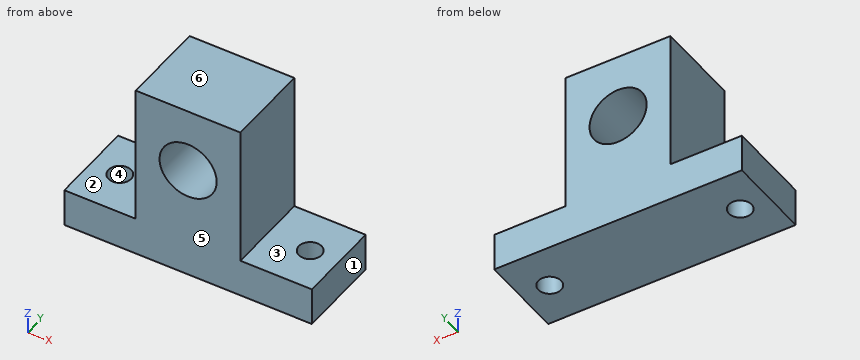
from build123d import *

# Parameters (mm, degrees)
F0_W     = 17.4625
F0_H     = 23.495
F0_R     = 4.7625
F1_DEPTH = 14.2875
F3_D     = 3.7973


with BuildPart() as f1:
    # F0 (on Front) → F1 (new body)
    with BuildSketch(Plane.XZ):
        with Locations((0, 14.9225)):
            Rectangle(F0_W, F0_H)
        with Locations((0, 15.875)):
            Circle(F0_R, mode=Mode.SUBTRACT)
        Polygon((20.6375, -3.175), (20.6375, 3.175), (8.73125, 3.175), (-8.73125, 3.175), (-20.6375, 3.175), (-20.6375, -3.175), align=None)
    extrude(amount=F1_DEPTH)

    # F3 (through all)
    with Locations(Plane(origin=(0, 0, -3.175), x_dir=(1, 0, 0), z_dir=(0, 0, -1))):
        with Locations((-15.875, 7.14375), (15.875, 7.14375)):
            Hole(F3_D / 2)


solid = f1.part
Can you work these out from the model? Positions are in its coordinate system, mm. Face numbers are marked on the shaded views. A direction names the side the tool comes from. Round coordinates to 2 decimals unless told otherwise and drop trailing zeros. Order: outer loops, then holes, each group sorted by start corner. A loop starts at its lowest first (then second) coordinate and runs counter-clockwise, first axis right, second up. Notation, with made-up numbers: (68.25, 53.5) - (119.25, 53.5) arc R16 cw to (119.25, 57.5) - close; hole circle Ø6 at (83, 25.5). An arc over 180 degrees is marked (long way). Answer in a Markdown table with one row per item.
(1) For P1, Ø1, axis at y = -7.5, z = 15.5, coming from the +X side, with a flat end and sliding along its axis, tell me the tip position at first contact or that it passes through.
From the geometry:
| item | result |
|---|---|
| P1 | stops at x = 8.73 |
(2) Suppose I cut it at C-C, the plane y = -11.75. Please give me the cut outline in (x, z) (1 decimal), plus the area to 3 significant figures.
From the geometry:
| item | result |
|---|---|
| outline | (-20.6, -3.2) - (20.6, -3.2) - (20.6, 3.2) - (8.7, 3.2) - (8.7, 26.7) - (-8.7, 26.7) - (-8.7, 3.2) - (-20.6, 3.2) - close; hole circle Ø9.5 at (0, 15.9) |
| area | 601 mm2 |
(3) Which directions (+Z, -Z, +X, -X, +Y, -Y) give clear straight access to the entire face, cutting with the end or side of a thin tool? Please do the marked faces 1, 2 and 3.
From the geometry:
| item | result |
|---|---|
| face 1 | +Z, -Z, +X, +Y, -Y |
| face 2 | +Z, -X, +Y, -Y |
| face 3 | +Z, +X, +Y, -Y |
(4) Suppose I cut it at B-B, the plane z = 14.75. Please give me the cut outline in (x, y).
From the geometry:
| item | result |
|---|---|
| outline | (-8.73, -14.29) - (-4.63, -14.29) - (-4.63, 0) - (-8.73, 0) - close; (4.63, -14.29) - (8.73, -14.29) - (8.73, 0) - (4.63, 0) - close |
(5) If we mould it in two halves opening along Y, with no side actions, what happens to the marked faces 4, 5 and 6? For each: released by +Y, released by -Y, zero draft, split by the parting line, or undercut.
From the geometry:
| item | result |
|---|---|
| face 4 | undercut |
| face 5 | released by -Y |
| face 6 | zero draft |
(6) Please list where these lines run through material, in increasing order: L1, parallel to Z at x = 0, y = -8.5 (1 decimal); L2, parallel to Z at x = -12, y = -4.75 (3 decimals); L3, parallel to X at y = -9.25, z = 3.25. Write a range as from..to.
From the geometry:
| item | result |
|---|---|
| L1 | z = -3.2..11.1, 20.6..26.7 |
| L2 | z = -3.175..3.175 |
| L3 | x = -8.73..8.73 |
(7) Suppose I cut it at D-D, the plane x = -12. Please give me the cut outline in (y, z) (1 decimal), plus the area to 3 significant figures.
From the geometry:
| item | result |
|---|---|
| outline | (-14.3, -3.2) - (0, -3.2) - (0, 3.2) - (-14.3, 3.2) - close |
| area | 90.7 mm2 |
(8) Suppose I cut it at A-A, the plane x = 0. Please give me the cut outline in (y, z) (1 decimal), plus the area to 3 significant figures.
From the geometry:
| item | result |
|---|---|
| outline | (-14.3, -3.2) - (0, -3.2) - (0, 11.1) - (-14.3, 11.1) - close; (-14.3, 20.6) - (0, 20.6) - (0, 26.7) - (-14.3, 26.7) - close |
| area | 290 mm2 |
